```python
from build123d import *

# Parameters (mm, degrees)
BOSS_EXTRUDE4_DEPTH = 50
SKETCH7_R           = 1.75
CUT_EXTRUDE1_DEPTH  = 17.825
SKETCH8_R           = 0.75
SKETCH8_W           = 11.8
SKETCH8_H           = 22.5
BOSS_EXTRUDE5_DEPTH = 6
SKETCH9_R           = 4.05
BOSS_EXTRUDE6_DEPTH = 8
FILLET1_R           = 3


with BuildPart() as part:
    # Sketch6 → Boss-Extrude4 (new body)
    with BuildSketch(Plane.XZ):
        with BuildLine():
            Line((-1, 25.784833184), (-1, 12.785954208))
            ThreePointArc((-1, 12.785954208), (-12.825, 0), (-1, -12.785954208))
            Line((-1, -12.785954208), (-1, -25.784833184))
            Line((-1, -25.784833184), (-6, -25.784833184))
            Line((-6, -25.784833184), (-6, -16.784833184))
            ThreePointArc((-6, -16.784833184), (-17.825, 0), (-6, 16.784833184))
            Line((-6, 16.784833184), (-6, 25.784833184))
            Line((-6, 25.784833184), (-1, 25.784833184))
        make_face()
    extrude(amount=BOSS_EXTRUDE4_DEPTH)

    # Sketch7 → Cut-Extrude1 (cut, through all)
    with BuildSketch(Plane(origin=(-1, 0, 0), x_dir=(0, 0, -1), z_dir=(1, 0, 0))):
        with Locations((-19.285393696, -10)):
            Circle(SKETCH7_R)
        with Locations((-19.285393696, -40)):
            Circle(SKETCH7_R)
        with Locations((19.285393696, -40)):
            Circle(SKETCH7_R)
        with Locations((19.285393696, -10)):
            Circle(SKETCH7_R)
    extrude(amount=-CUT_EXTRUDE1_DEPTH, mode=Mode.SUBTRACT)

    # Sketch8 → Boss-Extrude5 (add)
    with BuildSketch(Plane(origin=(0, 0, 0), x_dir=(1, 0, 0), z_dir=(0, 1, 0))):
        with BuildLine():
            Line((-32.320841509, -16.25), (-22.318992281, -16.25))
            ThreePointArc((-22.318992281, -16.25), (-21.069616181, -16.522536094), (-20.047240136, -17.290627093))
            ThreePointArc((-20.047240136, -17.290627093), (26.473715688, 0), (-20.047240136, 17.290627093))
            ThreePointArc((-20.047240136, 17.290627093), (-21.069616181, 16.522536094), (-22.318992281, 16.25))
            Line((-22.318992281, 16.25), (-32.320841509, 16.25))
            ThreePointArc((-32.320841509, 16.25), (-34.442161852, 15.371320344), (-35.320841509, 13.25))
            Line((-35.320841509, 13.25), (-35.320841509, -13.25))
            ThreePointArc((-35.320841509, -13.25), (-34.442161852, -15.371320344), (-32.320841509, -16.25))
        make_face()
        with Locations((-24.420841509, 13.65)):
            Circle(SKETCH8_R, mode=Mode.SUBTRACT)
        with Locations((-24.420841509, -13.65)):
            Circle(SKETCH8_R, mode=Mode.SUBTRACT)
        with Locations((-24.420841509, 0)):
            Rectangle(SKETCH8_W, SKETCH8_H, mode=Mode.SUBTRACT)
    extrude(amount=BOSS_EXTRUDE5_DEPTH)

    # Sketch9 → Boss-Extrude6 (add)
    with BuildSketch(Plane(origin=(0, 6, 0), x_dir=(1, 0, 0), z_dir=(0, 1, 0))):
        Circle(SKETCH9_R)
    extrude(amount=BOSS_EXTRUDE6_DEPTH)

    # Fillet1
    fillet1_edges = [part.edges().sort_by_distance(p)[0] for p in [
        (-4.05, 6, 0),
    ]]
    fillet(fillet1_edges, radius=FILLET1_R)


solid = part.part
```
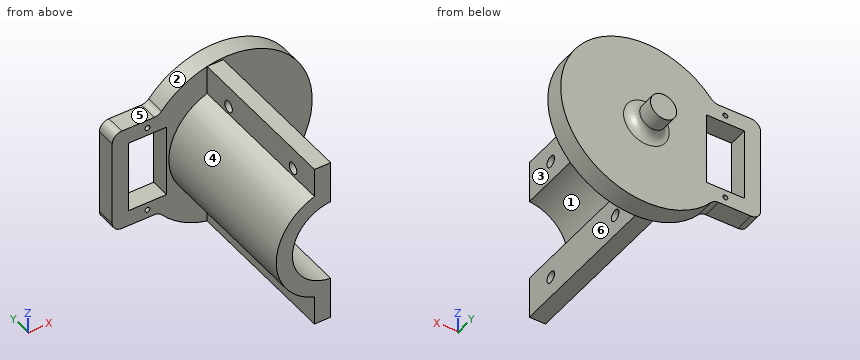
Geometry: final body of the model. Coordinates: model frame, mm. Face numbers are marked on the shaded views. A direction names the side the tool comes from. Coordinates: 2 decimals unless noted, no trailing zeros. Order: outer loops, then holes, each group sorted by start corner. A loop starts at its lowest first (then second) coordinate and runs counter-clockwise, first axis right, second up. Notation, with made-up numbers: M -18,-4.75 L 12,-4.75 A20 ccw 12,26.25 Z; hole C -20.75,81 d5. An arc over 180 degrees is marked long. Answer as CSV lines item,"result".
Q1. Section A-A on y = -10. Return the cut outline in (x, z) (3 decimals), and give its area (3 significant figures).
Answers:
outline,"M -6,-25.785 L -1,-25.785 L -1,-21.035 L -6,-21.035 Z; M -6,-17.535 L -1,-17.535 L -1,-12.786 A12.825 cw -1,12.786 L -1,17.535 L -6,17.535 L -6,16.785 A17.825 ccw -6,-16.785 Z; M -6,21.035 L -1,21.035 L -1,25.785 L -6,25.785 Z"
area,"279 mm^2"
Q2. Draft query along Z for the marked faces 1, 2 and 3. Return one class per face: pulls with the +Z half, pulls with the -Z half, needs draft (parallel to the pull), parting line crosses it, or undercut.
Answers:
face 1,"undercut"
face 2,"parting line crosses it"
face 3,"needs draft"
Q3. Section D-D on x = 0. Return the cut outline in (y, z).
Answers:
outline,"M 0,-26.47 L 6,-26.47 L 6,-7.05 A3 cw 9,-4.05 L 14,-4.05 L 14,4.05 L 9,4.05 A3 cw 6,7.05 L 6,26.47 L 0,26.47 Z"
Q4. Section C-C on y = 2.5. Return the cut outline in (x, z).
Answers:
outline,"M -35.32,-13.25 A3 ccw -32.32,-16.25 L -22.32,-16.25 A3 cw -20.05,-17.29 A26.47 ccw long -20.05,17.29 A3 cw -22.32,16.25 L -32.32,16.25 A3 ccw -35.32,13.25 Z; hole M -30.32,-11.25 L -18.52,-11.25 L -18.52,11.25 L -30.32,11.25 Z; hole C -24.42,-13.65 d1.5; hole C -24.42,13.65 d1.5"
Q5. First-contact query: P1, Ø7, axis at y = -20.5, z = 19.5, coming from the -X side; P2, Ø1.8, axis at x = -24, y = 2, coming from the -Z side; P3, Ø10, axis at x = -3, z = -19, coming from the +Y side. Flat tips, straight axial feed; report the tip coordinate or a pass-through.
Answers:
P1,"stops at x = -7.86"
P2,"stops at z = -16.25"
P3,"stops at y = 6"
Q6. Section B-B on z = 0. Return the cut outline in (x, y) (3 decimals).
Answers:
outline,"M -35.321,0 L -30.321,0 L -30.321,6 L -35.321,6 Z; M -18.521,0 L -17.825,0 L -17.825,-50 L -12.825,-50 L -12.825,0 L 26.474,0 L 26.474,6 L 7.05,6 A3 cw 4.05,9 L 4.05,14 L -4.05,14 L -4.05,9 A3 cw -7.05,6 L -18.521,6 Z"
Q7. Line query: probe 1 along X at (y, z) = (-45.5, -20.5); probe 2 along Y at (x, z) = (-12.5, 2); probe 3 along Y at (x, z) = (-6, 12.5). Output: solid intervals per line, ascending. Write a range as [from, to].
Answers:
probe 1,"x = [-6, -1]"
probe 2,"y = [0, 6]"
probe 3,"y = [-50, 6]"
Q8. Set-up query: the marked faces 4, 5 and 6. Return all of +Z, -Z, +X, -X, +Y, -Y with unobstructed straight access to the full face (end or side cutting, diameter ignored); none if empty.
Answers:
face 4,"-X, -Y"
face 5,"+Z, -X, +Y, -Y"
face 6,"+Z, -Z, +X, -Y"
